Geometry: final body of the model. Coordinates: model frame, mm. A direction names the side the tool comes from. Give positions to 0.01 mm unless a question says otherwise; leave off trailing zeros. Write each loop counter-clockwise with the first axis right and the second up, starting at its lowest first coordinate (ties: lowest second). Pieces come first, ordered by that corner, then holes. Notation, with made-up numbers: (49.5, 44) -> (102.5, 44) arc R4 ccw to (102.5, 49) -> close; hole circle Ø10 at (-2, -25.5). An arc over 180 degrees is marked (long way). Answer in a Markdown table with one row per item. Add a question column.
Item 1: Material intervals for probe 1 along X at (y, z) = (61.5, 0) (3 decimals); probe 2 along Z at (x, y) = (-2, 59.5); probe 3 along X at (y, z) = (57.5, 1.5), sorted ascending. Write a range as from..to.
Item 2: Section query A-A on z = 0. Output: boundary loops of the cut face in (x, y) (3 decimals).
Item 3: First-contact query: P1, Ø2, axis at x = -5.5, y = 79, coming from the -Z side (3 decimals); P2, Ø6, axis at x = 6.5, y = 2.5, coming from the +Z side; P3, Ø10, axis at x = 0, z = 0, coming from the -Y side; P4, Ø1.5, axis at x = 4, z = -4.5, coming from the -Y side. Flat tips, straight axial feed; report the tip coordinate or a pass-through.
Item 4: Draft query along X for faces 1 (the conical face through (-6.39, 82.5, -1.42)), 2 (the flat face through (-1.1, -12.7, 3.3)), 3 (the cylindrical face through (-1.93, 40.59, -2.52)). Return one class per face: +X half, -X half, draft (parallel to the pull), parting line (faces both ways), or undercut.
Item 5: Section query B-B on x = 0. Output: boundary loops of the cut face in (y, z) (3 decimals).
Item 6: Access query for faces 4 (the cylindrical face through (-3.86, 88.33, -5.04)), 5 (the cylindrical face through (-5.796, 40.814, -7.559)), 6 (the cylindrical face through (-3.86, -5.8, -5.04)). Directions: +Z, -Z, +X, -X, +Y, -Y. A direction counts if a zero-diameter tool reaches every point of the face in a straight line with its end or side. Return the directions, or none.
Item 7: Section query C-C on y = 34.5. Output: boundary loops of the cut face in (x, z) (3 decimals), plus the area to 3 significant figures.
```python
from build123d import *

# Parameters (mm, degrees)
SKETCH1_R           = 9.525
SKETCH1_R_2         = 3.175
SKETCH1_R_3         = 6.35
BOSS_EXTRUDE1_DEPTH = 82.69732
CHAMFER1_SIZE       = 3.175
BOSS_EXTRUDE2_START = -12.7
SKETCH1_3_R         = 6.35
SKETCH1_3_R_2       = 3.175
BOSS_EXTRUDE2_DEPTH = 12.7
BOSS_EXTRUDE3_START = 82.69732
SKETCH1_4_R         = 6.35
SKETCH1_4_R_2       = 3.175
BOSS_EXTRUDE3_DEPTH = 12.7
CHAMFER2_SIZE       = 1.27


with BuildPart() as part:
    # Sketch1 → Boss-Extrude1 (new body)
    # profile 1 of 2: a face of its own
    with BuildSketch(Plane(origin=(0, 0, 0), x_dir=(1, 0, 0), z_dir=(0, 1, 0))):
        with Locations(Location((0, 0, 0), (0, 0, 270))):
            Circle(SKETCH1_R)
        with Locations(Location((0, 0, 0), (0, 0, 270))):
            Circle(SKETCH1_R_2, mode=Mode.SUBTRACT)
    # profile 2 of 2: a face of its own
    with BuildSketch(Plane(origin=(0, 0, 0), x_dir=(1, 0, 0), z_dir=(0, 1, 0))):
        Circle(SKETCH1_R_3)
        with Locations(Location((0, 0, 0), (0, 0, 270))):
            Circle(SKETCH1_R_2, mode=Mode.SUBTRACT)
    extrude(amount=BOSS_EXTRUDE1_DEPTH)

    # Chamfer1
    chamfer1_edges = [part.edges().sort_by_distance(p)[0] for p in [
        (0, 0, -9.525),
        (0, 82.69732, -9.525),
    ]]
    chamfer(chamfer1_edges, length=CHAMFER1_SIZE)

    # Sketch1<3> → Boss-Extrude2 (add)
    with BuildSketch(Plane(origin=(0, 0, 0), x_dir=(1, 0, 0), z_dir=(0, 1, 0)).offset(BOSS_EXTRUDE2_START)):
        with Locations(Location((0, 0, 0), (0, 0, 270))):
            Circle(SKETCH1_3_R)
        with Locations(Location((0, 0, 0), (0, 0, 270))):
            Circle(SKETCH1_3_R_2, mode=Mode.SUBTRACT)
    extrude(amount=BOSS_EXTRUDE2_DEPTH)

    # Sketch1<4> → Boss-Extrude3 (add)
    with BuildSketch(Plane(origin=(0, 0, 0), x_dir=(1, 0, 0), z_dir=(0, 1, 0)).offset(BOSS_EXTRUDE3_START)):
        with Locations(Location((0, 0, 0), (0, 0, 270))):
            Circle(SKETCH1_4_R)
        with Locations(Location((0, 0, 0), (0, 0, 270))):
            Circle(SKETCH1_4_R_2, mode=Mode.SUBTRACT)
    extrude(amount=BOSS_EXTRUDE3_DEPTH)

    # Chamfer2
    chamfer2_edges = [part.edges().sort_by_distance(p)[0] for p in [
        (0, -12.7, -6.35),
        (0, 95.39732, -6.35),
    ]]
    chamfer(chamfer2_edges, length=CHAMFER2_SIZE)


solid = part.part
```
Findings below:
| question | item | result |
|---|---|---|
| 1 | probe 1 | x = -9.525..-3.175, 3.175..9.525 |
| 1 | probe 2 | z = -9.31..-2.47, 2.47..9.31 |
| 1 | probe 3 | x = -9.41..-2.8, 2.8..9.41 |
| 2 | outline | (-9.525, 3.175) -> (-6.35, 0) -> (-6.35, -11.43) -> (-5.08, -12.7) -> (-3.175, -12.7) -> (-3.175, 95.397) -> (-5.08, 95.397) -> (-6.35, 94.127) -> (-6.35, 82.697) -> (-9.525, 79.522) -> close; (3.175, -12.7) -> (5.08, -12.7) -> (6.35, -11.43) -> (6.35, 0) -> (9.525, 3.175) -> (9.525, 79.522) -> (6.35, 82.697) -> (6.35, 94.127) -> (5.08, 95.397) -> (3.175, 95.397) -> close |
| 3 | P1 | stops at z = -8.395 |
| 3 | P2 | stops at z = 8.83 |
| 3 | P3 | stops at y = -12.7 |
| 3 | P4 | stops at y = -12.51 |
| 4 | face 1 | parting line |
| 4 | face 2 | draft |
| 4 | face 3 | undercut |
| 5 | outline | (-12.7, -5.08) -> (-11.43, -6.35) -> (0, -6.35) -> (3.175, -9.525) -> (79.522, -9.525) -> (82.697, -6.35) -> (94.127, -6.35) -> (95.397, -5.08) -> (95.397, -3.175) -> (-12.7, -3.175) -> close; (-12.7, 3.175) -> (95.397, 3.175) -> (95.397, 5.08) -> (94.127, 6.35) -> (82.697, 6.35) -> (79.522, 9.525) -> (3.175, 9.525) -> (0, 6.35) -> (-11.43, 6.35) -> (-12.7, 5.08) -> close |
| 6 | face 4 | +Y |
| 6 | face 5 | +Y, -Y |
| 6 | face 6 | -Y |
| 7 | outline | circle Ø19.05 at (0, 0); hole circle Ø6.35 at (0, 0) |
| 7 | area | 253 mm^2 |
